Read the model definition and answer for the solid it produces. Units are mm, in the model's axes. A direction names the side the tool comes from. Coordinates: 2 decimals unless noted, no trailing zeros.
from build123d import *

# Parameters (mm, degrees)
SKETCH1_R           = 11
BOSS_EXTRUDE1_DEPTH = 3.5
SKETCH2_R           = 4.05
CUT_EXTRUDE3_DEPTH  = 6
CIRPATTERN1_COUNT   = 7


with BuildPart() as part:
    # Sketch1 → Boss-Extrude1 (new body, symmetric)
    with BuildSketch(Plane.XY):
        Polygon((-19.978492755, 0), (-12.456386489, -15.619814608), (4.445632867, -19.47759023), (18, -8.668343139), (18, 8.668343139), (4.445632867, 19.47759023), (-12.456386489, 15.619814608), align=None)
        Circle(SKETCH1_R, mode=Mode.SUBTRACT)
    extrude(amount=BOSS_EXTRUDE1_DEPTH, both=True)

    # Sketch2 → Cut-Extrude3 (cut)
    with BuildSketch(Plane(origin=(0.058998969, -18.476369669, 0), x_dir=(-0.974927912, 0.222520934, 0), z_dir=(-0.222520934, -0.974927912, 0))):
        with Locations((4.168898776, 0)):
            Circle(SKETCH2_R)
    cut_extrude3 = extrude(amount=-CUT_EXTRUDE3_DEPTH, mode=Mode.SUBTRACT)

    # CirPattern1: Cut-Extrude3 ×7 about axis
    cirpattern1_axis = Axis((0, 0, 0), (0, 0, 1))
    for i in range(1, CIRPATTERN1_COUNT):
        add(cut_extrude3.rotate(cirpattern1_axis, i * 360 / CIRPATTERN1_COUNT), mode=Mode.SUBTRACT)


solid = part.part
Item 1: Which of the six approach directions +Z, -Z, +X, -X, +Y, -Y give full straight-line access (tool end or side, diameter ignored) to faces 1 (the face through (-15.31, 2.88, -0.06)), 2 (the face through (15.04, 4.05, -0.06)), 3 (the face through (-9.897, 16.204, 0.049)), 4 (the face through (6.425, -17.899, 0.049)), 5 (the face through (-11.795, 10.175, 0.059))?
Numbers:
face 1: none
face 2: +X
face 3: +Z, -Z, -X, +Y
face 4: +Z, -Z, +X, -Y
face 5: -X
Item 2: Given pin 1 (3.5 mm diameter, centred on y = -1, z = 1.5, fed in from +X); pin 2 (3 mm diameter, centred on x = -1, z = -1.5, fed in from +Y), each flat-ended and moving along its own axis, determine where each tip first touches the part or whether it passes through.
Numbers:
pin 1: stops at x = 12
pin 2: stops at y = 18.58
Item 3: A cutting plane is placed at A-A on y = 2.5. Give the number of separate pieces and of enclosed holes in the cut face, then the cut area to 3 significant figures.
Numbers:
separate pieces: 2
enclosed holes: 1
area: 60.2 mm2
Item 4: Determine the mould class of faces 6 (the face through (-13.555, 13.338, 0.049)), 7 (the face through (-15.31, -2.88, 0.06)), 8 (the face through (18, -6, 0)) for opening direction Y: released by +Y, released by -Y, zero draft, split by the parting line, or undercut.
Numbers:
face 6: released by +Y
face 7: undercut
face 8: zero draft
Item 5: Find the intervals of material crossed by line 1 along Y through (x, z) = (-12, -1.5); line 2 along X through (y, z) = (4, 1.25); line 3 along X through (y, z) = (-1.5, 2.75), in increasing order.
Numbers:
line 1: y = -15.72 to -9.95, -2.74 to 2.74, 9.95 to 15.72
line 2: x = -18.05 to -17.18, -11.39 to -10.25, 10.25 to 18
line 3: x = -19.26 to -10.9, 10.9 to 12
